from build123d import *

# Parameters (mm, degrees)
EXTRUDE_1_DEPTH  = 5.6
SKETCH_3_W       = 20
SKETCH_3_H       = 10
EXTRUDE_2_DEPTH  = 2.5
EXTRUDE_3_REACH  = 77.491
EXTRUDE_4_DEPTH  = 2.5
SKETCH_7_W       = 28.4
SKETCH_7_H       = 17.12
EXTRUDE_5_DEPTH  = 4.9
SKETCH_8_W       = 39.9
SKETCH_8_H       = 17.12
EXTRUDE_6_DEPTH  = 2.5
SKETCH_9_W       = 17.5
SKETCH_9_H       = 15
EXTRUDE_7_DEPTH  = 2.5
EXTRUDE_8_DEPTH  = 19.9
FILLET_1_R       = 1
EXTRUDE_9_REACH  = 103.831
SKETCH_14_W      = 4.8
SKETCH_14_H      = 30
EXTRUDE_12_DEPTH = 83.9
EXTRUDE_13_DEPTH = 8.56
FILLET_3_R       = 1


with BuildPart() as part:
    # Sketch 1 → Extrude 1 (new body)
    with BuildSketch(Plane.XY):
        Polygon((0, 49.365), (5, 54.365), (45, 54.365), (50, 49.365), (50, 0), (0, 0), align=None)
    extrude(amount=EXTRUDE_1_DEPTH)

    # Sketch 5 → Extrude 3 (add, up to next)
    with BuildSketch(Plane(origin=(0, 0, 15.6), x_dir=(-1, 0, 0), z_dir=(0, 0, -1)), mode=Mode.PRIVATE) as extrude_3_sk1:
        Polygon((-30, 43.145), (-50, 40.645), (-50, 38.145), (-30, 38.145), align=None)
    extrude_3_tool1 = extrude(extrude_3_sk1.sketch, amount=EXTRUDE_3_REACH, mode=Mode.PRIVATE) - part.part


with BuildPart() as body_2:
    # Sketch 3 → Extrude 2 (new body)
    with BuildSketch(Plane.XY.offset(15.6)):
        with Locations((40, 43.145)):
            Rectangle(SKETCH_3_W, SKETCH_3_H)
    extrude(amount=EXTRUDE_2_DEPTH)


with BuildPart() as part_1:
    add(part.part)

    add(body_2.part)  # Extrude 3 merges body 2
    add(extrude_3_tool1.solids().sort_by_distance((38.888889, 40.089444, 15.6))[0])

    # Sketch 6 → Extrude 4 (add)
    with BuildSketch(Plane.ZY.offset(-30)):
        Polygon((18.1, 43.145), (70.1, 15), (70.1, 0), (5.6, 0), (5.6, 38.145), (18.1, 38.145), align=None)
    extrude(amount=-EXTRUDE_4_DEPTH)

    # Sketch 9 → Extrude 7 (add)
    with BuildSketch(Plane.XY.offset(70.1)):
        with Locations((41.25, 7.5)):
            Rectangle(SKETCH_9_W, SKETCH_9_H)
    extrude(amount=-EXTRUDE_7_DEPTH)



with BuildPart() as body_2_2:
    # Sketch 7 → Extrude 5 (new body)
    with BuildSketch(Plane.ZY.offset(-5.2)):
        with Locations((75.3, 8.56)):
            Rectangle(SKETCH_7_W, SKETCH_7_H)
    extrude(amount=-EXTRUDE_5_DEPTH)

    # Sketch 8 → Extrude 6 (add)
    with BuildSketch(Plane.XY.offset(89.5)):
        with Locations((30.05, 8.56)):
            Rectangle(SKETCH_8_W, SKETCH_8_H)
    extrude(amount=-EXTRUDE_6_DEPTH)


with BuildPart() as part_2:
    add(part_1.part)

    add(body_2_2.part)  # Extrude 8 merges body 2 2
    # Sketch 11 → Extrude 8 (add)
    with BuildSketch(Plane(origin=(10.1, 0, 0), x_dir=(0, 0, -1), z_dir=(1, 0, 0))):
        Polygon((-61.1, 0), (-61.1, 7), (-70.1, 8.56), (-87, 8.56), (-87, 0), align=None)
    extrude(amount=EXTRUDE_8_DEPTH)

    # Fillet 1
    fillet_1_edges = [part_2.edges().sort_by_distance(p)[0] for p in [
        (20.05, 7, 61.1),
    ]]
    fillet(fillet_1_edges, radius=FILLET_1_R)

    # Sketch 12 → Extrude 9 (add, up to next)
    with BuildSketch(Plane.XY.offset(70.1), mode=Mode.PRIVATE) as extrude_9_sk1:
        Polygon((30, 0), (30, 8.56), (50, 11), (50, 0), align=None)
    extrude_9_tool1 = extrude(extrude_9_sk1.sketch, amount=EXTRUDE_9_REACH, mode=Mode.PRIVATE) - part_2.part
    add(extrude_9_tool1.solids().sort_by_distance((40.415815, 4.915365, 70.1))[0])

    # Sketch 14 → Extrude 12 (add)
    with BuildSketch(Plane.XY.offset(5.6)):
        with Locations((2.4, 15)):
            Rectangle(SKETCH_14_W, SKETCH_14_H)
    extrude(amount=EXTRUDE_12_DEPTH)

    # Sketch 15 → Extrude 13 (add)
    with BuildSketch(Plane(origin=(0, 8.56, 0), x_dir=(1, 0, 0), z_dir=(0, 1, 0))):
        with BuildLine():
            Line((10.1, -79.5), (10.1, -87))
            Line((10.1, -87), (17.6, -87))
            ThreePointArc((17.6, -87), (12.296699141, -84.803300859), (10.1, -79.5))
        make_face()
    extrude(amount=EXTRUDE_13_DEPTH)

    # Fillet 3
    # the kernel refuses this fillet: 1 mm, written as the material it takes off along each edge
    with BuildSketch(Plane(origin=(30, 17.5, 70.1), x_dir=(0, 0, -1), z_dir=(0, -1, 0))) as fillet_3_piece_1_section:
        with BuildLine():
            CenterArc((FILLET_3_R, FILLET_3_R), FILLET_3_R, 180, 90)
            Line((0, FILLET_3_R), (0, 0))
            Line((0, 0), (FILLET_3_R, 0))
        make_face()
    fillet_3_piece_1 = extrude(amount=11.44, mode=Mode.PRIVATE)
    fillet_3_piece_1 = split(fillet_3_piece_1, bisect_by=Plane(origin=(30.761446194, 8.652896436, 69.873228865), z_dir=(-0.12110208706144665, 0.9926400578806811, 0)), keep=Keep.TOP, mode=Mode.PRIVATE)
    add(fillet_3_piece_1, mode=Mode.SUBTRACT)


solid = part_2.part
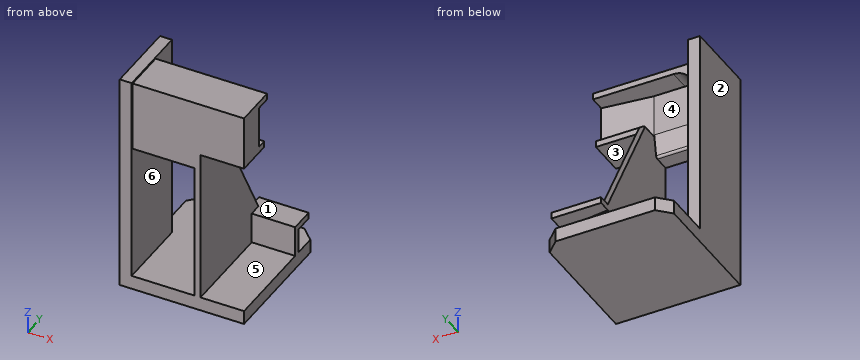
Design review of the part built by this model. Coordinates are the model's own, in mm. Face numbers are marked on the shaded views. A direction names the side the tool comes from. Give positions to 0.01 mm unless a question says otherwise; leave off trailing zeros. Order: outer loops, then holes, each group sorted by start corner. A loop starts at its lowest first (then second) coordinate and runs counter-clockwise, first axis right, second up.
1. Tool access review of the marked faces 4, 5 and 6: name each direction out of +Z, -Z, +X, -X, +Y, -Y from which nothing blocks a thin tool from reaching the whole face with its end or side.
Solution:
face 4: +Y
face 5: +X, -Y
face 6: +Z, +Y, -Y
2. Add section B-B, the plane x = 29. State the section outline as (y, z) points (3 decimals), then the cut area to 3 significant figures.
Solution:
outline: (0, 0) - (54.365, 0) - (54.365, 5.6) - (0, 5.6) - close; (0, 61.1) - (6.158, 61.1) arc R1 ccw to (7.144, 61.929) - (8.56, 70.1) - (8.56, 87) - (17.12, 87) - (17.12, 89.5) - (0, 89.5) - close
area: 562 mm2
3. To check wall thickness, follow L1, parallel to Z at x = 44, y = 12; L2, parallel to X at y = 4, z = 20.5; L3, parallel to Z at x = 10, y = 7.5. State the ranges of each line that lie inside material, in increasing order.
Solution:
L1: z = 0 to 5.6, 67.6 to 70.1, 87 to 89.5
L2: x = 0 to 4.8, 30 to 32.5
L3: z = 0 to 5.6, 61.1 to 89.5
4. Add section C-C, the plane y = 4. State the section outline as (x, z) points.
Solution:
outline: (0, 0) - (50, 0) - (50, 5.6) - (32.5, 5.6) - (32.5, 67.6) - (50, 67.6) - (50, 89.5) - (5.2, 89.5) - (5.2, 61.1) - (30, 61.1) - (30, 5.6) - (4.8, 5.6) - (4.8, 89.5) - (0, 89.5) - close
5. Add section A-A, the plane z = 9. State the section outline as (x, y) points (3 decimals).
Solution:
outline: (0, 0) - (4.8, 0) - (4.8, 30) - (0, 30) - close; (30, 0) - (32.5, 0) - (32.5, 38.145) - (50, 38.145) - (50, 40.645) - (30, 43.145) - close
6. Mouldability with a two-part tool opening along Z and no side actions: class the marked faces 1, 2 and 3 as +Z half, -Z half, draft (parallel to the pull), parting line (faces both ways), or undercut.
Solution:
face 1: +Z half
face 2: draft
face 3: undercut
7. Add section D-D, the plane z = 84. State the section outline as (x, y) points.
Solution:
outline: (0, 0) - (4.8, 0) - (4.8, 30) - (0, 30) - close; (5.2, 0) - (50, 0) - (50, 11) - (30, 8.56) - (11.6, 8.56) - (11.6, 17.12) - (5.2, 17.12) - close
8. For pin 1 Ø5 at (x, y) = (40.5, 43.5) entering from +Z; pin 2 Ø8 at (x, z) = (36, 66.5) entering from +Y; pin 3 Ø1 at (x, z) = (14.5, 77.5) entering from +Y, all flat-tipped, find the tip position at first contact; note any pin that passes through.
Solution:
pin 1: stops at z = 18.1
pin 2: stops at y = 18
pin 3: stops at y = 8.56
